Answer from the drawing. Dimensions are ordinates in mm from the lowest x, y and z of the part. Coordinates: 2 decimals unless noted, no trailing zeros. Write each loop counter-clockwise with the first axis right and the second up, starting at its lowest first coordinate (ties: lowest second). Pieces come first, ordered by that corner, then holes.
(1) Section C-C on x = 2.75 is taken. Write down the section's boundary in (y, z).
(2) Section A-A on x = 15 is taken. Write down the section's boundary in (y, z) (1 decimal).
(3) Find the intervals of material crossed by probe 1 along Y at (x, z) = (15, 1.2) (1 decimal); probe 2 along X at (y, z) = (10.5, 2.8) (1 decimal); probe 3 along Y at (x, z) = (14, 1.75) (1 decimal), in increasing order.
(4) Section B-B on z = 2.9 is taken. Write down the section's boundary in (x, y) (1 decimal).
(5) Given pin 1 (1 mm diameter, centred on y = 20.5, z = 3.5, fed in from +X); pin 2 (2 mm diameter, centred on x = 8, z = 2, fed in from -Y), each flat-ended and moving along its own axis, determine where each tip first touches the part or whether it passes through.
(6) The mould has two halves that part along X. Classify the marked faces 1, 2 and 3: +X half, -X half, draft (parallel to the pull), parting line (faces both ways), or undercut.
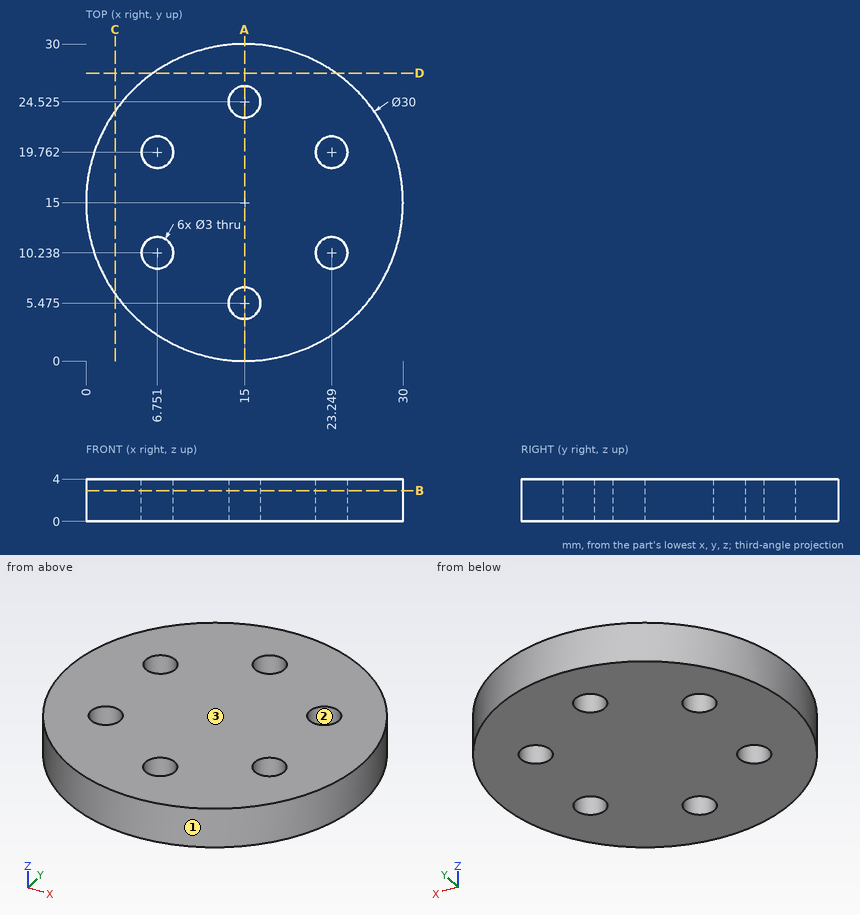
Response:
1. outline: (6.34, 0) - (23.66, 0) - (23.66, 4) - (6.34, 4) - close
2. outline: (0, 0) - (4, 0) - (4, 4) - (0, 4) - close; (7, 0) - (23, 0) - (23, 4) - (7, 4) - close; (26, 0) - (30, 0) - (30, 4) - (26, 4) - close
3. probe 1: y = 0 to 4, 7 to 23, 26 to 30
3. probe 2: x = 0.7 to 5.3, 8.2 to 21.8, 24.7 to 29.3
3. probe 3: y = 0 to 4.4, 6.6 to 23.4, 25.6 to 30
4. outline: circle Ø30 at (15, 15); hole circle Ø3 at (6.8, 10.2); hole circle Ø3 at (6.8, 19.8); hole circle Ø3 at (15, 5.5); hole circle Ø3 at (15, 24.5); hole circle Ø3 at (23.2, 10.2); hole circle Ø3 at (23.2, 19.8)
5. pin 1: stops at x = 29.14
5. pin 2: stops at y = 1.25
6. face 1: parting line
6. face 2: undercut
6. face 3: draft
